```python
from build123d import *

# Parameters (mm, degrees)
F0_R      = 1.75
F1_DEPTH  = 1.6
F2_W      = 7
F2_H      = 10.2
F3_DEPTH  = 8.5
F4_W      = 6.2
F4_H      = 6.2
F5_DEPTH  = 5.4
F6_R      = 1.725
F7_R      = 1.725
F8_DEPTH  = 0.6
F10_DEPTH = 1.5


with BuildPart() as f1:
    # F0 (on Top) → F1 (new body)
    with BuildSketch(Plane.XY):
        Polygon((-16.15, 5.1), (-23.15, 5.1), (-23.15, -5.1), (-16.15, -5.1), (-11.85, -7), (23.15, -7), (23.15, 7), (-11.85, 7), align=None)
        with Locations((-14.15, 0)):
            Circle(F0_R, mode=Mode.SUBTRACT)
    extrude(amount=F1_DEPTH)

    # F2 (on face) → F3 (join)
    with BuildSketch(Plane.XY.offset(1.6)):
        with Locations((-19.65, 0)):
            Rectangle(F2_W, F2_H)
    extrude(amount=F3_DEPTH)

    # F4 (on face) → F5 (join)
    with BuildSketch(Plane.XY.offset(1.6)):
        with Locations((-4.65, 0)):
            Rectangle(F4_W, F4_H)
        with Locations((10.95, 0)):
            Rectangle(F4_W, F4_H)
    extrude(amount=F5_DEPTH)

    # F6 (on face) + F7 (on face) → F8 (join)
    with BuildSketch(Plane.XY.offset(7)):
        with Locations((-4.65, 0)):
            Circle(F6_R)
    with BuildSketch(Plane.XY.offset(7)):
        with Locations((10.95, 0)):
            Circle(F7_R)
    extrude(amount=F8_DEPTH)

    # F9 (on face) → F10 (join)
    with BuildSketch(Plane(origin=(0, 0, 0), x_dir=(1, 0, 0), z_dir=(0, 0, -1))):
        Polygon((23.35, 7), (23.15, 7), (13.15, 7), (13.15, -7), (23.15, -7), (23.35, -7), align=None)
    extrude(amount=F10_DEPTH)


solid = f1.part
```
Verification items for the finished model (mm, model axes). A direction names the side the tool comes from. Coordinates: 2 decimals unless noted, no trailing zeros. Write each loop counter-clockwise with the first axis right and the second up, starting at its lowest first coordinate (ties: lowest second). Pieces come first, ordered by that corner, then holes. Notation, with made-up numbers: M -18,48 L 27,48 A25 ccw 27,71 Z; hole C 4,-0.75 d11. An arc over 180 degrees is marked long. Answer as a JSON object with one key per item and string values. Group by question number.
(1) Cross-section at D-D, the plane x = -2. Record the cut outline in (y, z), and give its area (3 significant figures).
(2) Cross-section at C-C, the plane y = 2.5. Record the cut outline in (x, z), and give its area (3 significant figures).
(3) Cross-section at A-A, the plane z = 5.75. Record the cut outline in (x, y).
(4) Release check for a two-part mould opening along X. For faces 1 (the face through (-13.97, 6.063, 0.789)), 2 (the face through (23.15, 0, 1)), 3 (the face through (-16.15, 0, 6)) record: +X half, -X half, draft (parallel to the pull), parting line (faces both ways), or undercut.
(5) Tool access check on faces 4 (the face through (-5, -3.1, 4)), 5 (the face through (13.15, 0, -1)), 6 (the face through (9.5, -1.3, 7)), 7 (the face through (11, 0, 7.6)), 8 (the face through (-7.75, 0, 4)). Record the directions out of +Z, -Z, +X, -X, +Y, -Y that give a thin tool (end or side, any length) a straight path to the whole face; none if there is none.
(6) Material ranges on line 1 (Z direction, x = -12.5, y = -3.5); line 2 (X direction, y = 4.5, z = 7.75); line 3 (Y direction, x = -14.15, z = 1.3), recorded low to high.
(7) Cross-section at B-B, the plane x = -14.15. Record the cut outline in (y, z), and give its area (3 significant figures).
(8) Gauge pin test, flat ends, axial feed: pin 1 (1 mm diameter, centred on x = -18, z = 5, fed in from +Y); pin 2 (6 mm diameter, centred on y = 1, z = 3.5, fed in from +X); pin 3 (5 mm diameter, centred on x = 10.5, y = 1, fed in from +Z); pin 4 (6 mm diameter, centred on x = -6, z = 4, fed in from +Y). Record the tip position at first contact, or that the pin passes through.
Reply:
{
 "1": {"outline": "M -7,0 L 7,0 L 7,1.6 L 3.1,1.6 L 3.1,7 L -3.1,7 L -3.1,1.6 L -7,1.6 Z", "area": "55.9 mm²"},
 "2": {"outline": "M -23.15,0 L 13.15,0 L 13.15,-1.5 L 23.35,-1.5 L 23.35,0 L 23.15,0 L 23.15,1.6 L 14.05,1.6 L 14.05,7 L 7.85,7 L 7.85,1.6 L -1.55,1.6 L -1.55,7 L -7.75,7 L -7.75,1.6 L -16.15,1.6 L -16.15,10.1 L -23.15,10.1 Z", "area": "216 mm²"},
 "3": {"outline": "M -23.15,-5.1 L -16.15,-5.1 L -16.15,5.1 L -23.15,5.1 Z; M -7.75,-3.1 L -1.55,-3.1 L -1.55,3.1 L -7.75,3.1 Z; M 7.85,-3.1 L 14.05,-3.1 L 14.05,3.1 L 7.85,3.1 Z"},
 "4": {"face 1": "-X half", "face 2": "+X half", "face 3": "undercut"},
 "5": {"face 4": "+Z, +X, -Y", "face 5": "-Z, -X, +Y, -Y", "face 6": "+Z", "face 7": "+Z, +X, +Y, -Y", "face 8": "+Z, +Y, -Y"},
 "6": {"line 1": "0 to 1.6", "line 2": "-23.15 to -16.15", "line 3": "-5.98 to -1.75, 1.75 to 5.98"},
 "7": {"outline": "M -5.98,0 L -1.75,0 L -1.75,1.6 L -5.98,1.6 Z; M 1.75,0 L 5.98,0 L 5.98,1.6 L 1.75,1.6 Z", "area": "13.5 mm²"},
 "8": {"pin 1": "y = 5.1", "pin 2": "x = 23.15", "pin 3": "z = 7.6", "pin 4": "y = 7"}
}
